from build123d import *

# Parameters (mm, degrees)
SKETCH2_W           = 9.52
SKETCH2_H           = 28.42
SKETCH2_W_2         = 3.01
SKETCH2_H_2         = 6
BOSS_EXTRUDE1_DEPTH = 10
SKETCH4_R           = 1.852493383
SKETCH4_R_2         = 1.85249338
CUT_EXTRUDE1_DEPTH  = 9.5


with BuildPart() as part:
    # Sketch2 → Boss-Extrude1 (new body)
    with BuildSketch(Plane.XY):
        with BuildLine():
            Line((0, 66.651771766), (0, 33.391771766))
            Line((0, 33.391771766), (-16.03, 33.391771766))
            ThreePointArc((-16.03, 33.391771766), (-16.53, 32.891771766), (-16.03, 32.391771766))
            Line((-16.03, 32.391771766), (1.352234191, 32.391771766))
            Line((1.352234191, 32.391771766), (1.352234191, 34.518218659))
            ThreePointArc((1.352234191, 34.518218659), (1.506462672, 34.749146821), (1.77885672, 34.695149386))
            Line((1.77885672, 34.695149386), (4.496782459, 31.98195805))
            ThreePointArc((4.496782459, 31.98195805), (4.727391952, 30.826554208), (3.747902937, 30.171771766))
            Line((3.747902937, 30.171771766), (3.470297616, 30.171771766))
            ThreePointArc((3.470297616, 30.171771766), (0.641870491, 29.00019889), (-0.529702384, 26.171771766))
            Line((-0.529702384, 26.171771766), (-0.529702384, 21.208235908))
            ThreePointArc((-0.529702384, 21.208235908), (-0.633785571, 20.193347464), (-0.941701806, 19.220712149))
            Line((-0.941701806, 19.220712149), (-5.050790824, 9.735289546))
            ThreePointArc((-5.050790824, 9.735289546), (-5.788270464, 8.858470858), (-6.885991056, 8.53029905))
            Line((-6.885991056, 8.53029905), (-9.79055056, 8.53029905))
            ThreePointArc((-9.79055056, 8.53029905), (-11.527191752, 9.538292312), (-11.513310325, 11.546221681))
            Line((-11.513310325, 11.546221681), (-6.265893795, 20.444574564))
            ThreePointArc((-6.265893795, 20.444574564), (-5.74917957, 21.668040962), (-5.572793209, 22.984381141))
            Line((-5.572793209, 22.984381141), (-5.572793209, 25.171771766))
            ThreePointArc((-5.572793209, 25.171771766), (-7.037259303, 28.707305672), (-10.572793209, 30.171771766))
            Line((-10.572793209, 30.171771766), (-21.54, 30.171771766))
            ThreePointArc((-21.54, 30.171771766), (-22.247106781, 30.464664985), (-22.54, 31.171771766))
            Line((-22.54, 31.171771766), (-22.54, 32.942649485))
            ThreePointArc((-22.54, 32.942649485), (-22.832893219, 33.649756266), (-23.54, 33.942649485))
            Line((-23.54, 33.942649485), (-23.98462025, 33.942649485))
            ThreePointArc((-23.98462025, 33.942649485), (-25.801884678, 34.695385057), (-26.55462025, 36.512649485))
            Line((-26.55462025, 36.512649485), (-26.55462025, 44.391771766))
            ThreePointArc((-26.55462025, 44.391771766), (-25.801884678, 46.209036193), (-23.98462025, 46.961771766))
            Line((-23.98462025, 46.961771766), (-23.54, 46.961771766))
            ThreePointArc((-23.54, 46.961771766), (-22.832893219, 47.254664985), (-22.54, 47.961771766))
            Line((-22.54, 47.961771766), (-22.54, 67.401771766))
            ThreePointArc((-22.54, 67.401771766), (-22.832893219, 68.108878547), (-23.54, 68.401771766))
            Line((-23.54, 68.401771766), (-23.98462025, 68.401771766))
            ThreePointArc((-23.98462025, 68.401771766), (-25.801884678, 69.154507338), (-26.55462025, 70.971771766))
            Line((-26.55462025, 70.971771766), (-26.55462025, 77.401771766))
            Line((-26.55462025, 77.401771766), (-26.55462025, 79.000903717))
            ThreePointArc((-26.55462025, 79.000903717), (-25.801884678, 80.818168145), (-23.98462025, 81.570903717))
            Line((-23.98462025, 81.570903717), (-20.021565093, 81.570903717))
            ThreePointArc((-20.021565093, 81.570903717), (-18.905624991, 81.31597989), (-18.011069886, 80.601781295))
            Line((-18.011069886, 80.601781295), (-17.190935487, 79.571798553))
            ThreePointArc((-17.190935487, 79.571798553), (-12.815621218, 76.078617097), (-7.357501728, 74.831771766))
            Line((-7.357501728, 74.831771766), (0.623852111, 74.831771766))
            ThreePointArc((0.623852111, 74.831771766), (2.441116539, 74.079036193), (3.193852111, 72.261771766))
            Line((3.193852111, 72.261771766), (3.193852111, 64.016682225))
            ThreePointArc((3.193852111, 64.016682225), (2.79053513, 63.543838386), (2.26, 63.867533241))
            Line((2.26, 63.867533241), (1.347357771, 66.651771766))
            Line((1.347357771, 66.651771766), (0, 66.651771766))
        make_face()
        with Locations((-11.27, 54.111771766)):
            Rectangle(SKETCH2_W, SKETCH2_H, mode=Mode.SUBTRACT)
        with Locations((-20.2649024, 75.392647139)):
            Rectangle(SKETCH2_W_2, SKETCH2_H_2, mode=Mode.SUBTRACT)
        with Locations((-20.2649024, 40.392647139)):
            Rectangle(SKETCH2_W_2, SKETCH2_H_2, mode=Mode.SUBTRACT)
    extrude(amount=BOSS_EXTRUDE1_DEPTH)

    # Sketch4 → Cut-Extrude1 (cut)
    with BuildSketch(Plane.ZY.offset(26.55462025)):
        with Locations((5, 75.452210625)):
            Circle(SKETCH4_R)
        with Locations((5, 40.452210625)):
            Circle(SKETCH4_R_2)
    extrude(amount=-CUT_EXTRUDE1_DEPTH, mode=Mode.SUBTRACT)


solid = part.part
The model under review builds one solid part; all positions refer to its coordinate system, in mm. A direction names the side the tool comes from. Round coordinates to 2 decimals unless told otherwise and drop trailing zeros. Loops run counter-clockwise (first coordinate to the right, second up) from the corner with the lowest first, then second, coordinate; pieces in that order, holes last. Notation, with made-up numbers: (-2, 19) -> (43, 19) arc R29 cw to (43, 40) -> close; hole circle Ø8 at (73.5, -20.75). An arc over 180 degrees is marked (long way). Write item = value, one per line. Start each with the question number.
Item 1: Take a section at B-B on x = -15. Give the boundary of the cut face in (y, z).
Item 2: For faces 5 (the cylindrical face through (-24.196, 73.809, 5.855)), 6 (the cylindrical face through (-5.754, 21.65, 4.93)), 7 (the flat face through (1.352, 33, 5)), 8 (the flat face through (-0.53, 24, 5)), list the 3-axis set-ups (+Z, -Z, +X, -X, +Y, -Y) from which the entire face can be reached by the end or side of a thin tool; tool diameter is ignored.
Item 3: Insertion check: pin 1 (1 mm diameter, centred on x = -18.5, z = 5.5, fed in from -Y); pin 2 (1.7 mm diameter, centred on y = 33.5, z = 6, fed in from -X); pin 3 (3 mm diameter, centred on y = 41.5, z = 3, fed in from +X). Each pin has a flat end and moves straight along its axis. Give the tip position at first contact, or say it passes through.
Item 4: To check wall thickness, follow L1, parallel to Y at x = -23.9, z = 5; L2, parallel to Y at x = -20, z = 3; L3, parallel to X at y = 48, z = 8. State the ranges of each line that lie inside material, in increasing order.
Item 5: Take a section at C-C on z = 7.75. Count the separate pieces of the cut face and the enclosed holes in it, plus the area to 3 significant figures.
Item 6: Take a section at A-A on x = -4. Give the boundary of the cut face in (y, z), plus the area to 3 significant figures.
Item 7: Take a section at D-D on y = 24.5. Give the boundary of the cut face in (x, z), plus the area to 3 significant figures.
Item 8: Mouldability with a two-part tool opening along Y and no side actions: class faces 1 (the cylindrical face through (-0.63, 20.21, 4.93)), 2 (the cylindrical face through (-25.82, 80.8, 4.93)), 3 (the flat face through (-26.555, 73, 5)), 4 (the cylindrical face through (-25.82, 46.19, 4.93)) as released by +Y, released by -Y, zero draft, split by the parting line, or undercut.
Result:
q1.outline = (30.17, 0) -> (32.39, 0) -> (32.39, 10) -> (30.17, 10) -> close; (33.39, 0) -> (39.9, 0) -> (39.9, 10) -> (33.39, 10) -> close; (68.32, 0) -> (77.42, 0) -> (77.42, 10) -> (68.32, 10) -> close
q2.face_5 = -X
q2.face_6 = +Z, -Z, -X
q2.face_7 = +Z, -Z
q2.face_8 = +Z, -Z, +X, -Y
q3.pin_1 = 30.17
q3.pin_2 = -25.37
q3.pin_3 = 0
q4.L1 = 33.94 to 38.6, 42.3 to 46.96, 68.4 to 73.6, 77.3 to 81.57
q4.L2 = 30.17 to 37.39, 43.39 to 72.39, 78.39 to 81.57
q4.L3 = -22.54 to -16.03, -6.51 to 0
q5.separate_pieces = 1
q5.enclosed_holes = 3
q5.area = 1,010 mm²
q6.outline = (12.16, 0) -> (32.39, 0) -> (32.39, 10) -> (12.16, 10) -> close; (33.39, 0) -> (74.83, 0) -> (74.83, 10) -> (33.39, 10) -> close
q6.area = 617 mm²
q7.outline = (-5.57, 0) -> (-0.53, 0) -> (-0.53, 10) -> (-5.57, 10) -> close
q7.area = 50.4 mm²
q8.face_1 = released by -Y
q8.face_2 = released by +Y
q8.face_3 = zero draft
q8.face_4 = undercut
